from build123d import *

# Parameters (mm, degrees)
SKETCH_395_R           = 7.6
EXTRUDE_923_DEPTH      = 15
CUT_EXTRUDE_1359_DEPTH = 10
SKETCH_4236_W          = 30
SKETCH_4236_H          = 12
SKETCH_4236_R          = 2.15
SKETCH_4236_R_2        = 4.1
EXTRUDE_5757_DEPTH     = 15
SKETCH_1_3_R           = 12.15
SKETCH_1_3_R_2         = 10.65
CUT_EXTRUDE_5889_DEPTH = 5
SKETCH_1_4_R           = 10.65
CUT_EXTRUDE_5977_DEPTH = 8.5
CUT_EXTRUDE_7570_DEPTH = 6
SKETCH_1_R             = 7.65
EXTRUDE_7865_DEPTH     = 6.5


with BuildPart() as part:
    # Sketch 395 → Extrude 923 (new body)
    with BuildSketch(Plane.XY):
        with BuildLine():
            Line((33.023854242, 2.889212872), (32.0215632, 14.3454519))
            Line((32.0215632, 14.3454519), (35.508244643, 14.650497))
            Line((35.508244643, 14.650497), (33.329351075, 39.555364452))
            Line((33.329351075, 39.555364452), (56.241829131, 41.559946535))
            Line((56.241829131, 41.559946535), (58.4207227, 16.655079083))
            Line((58.4207227, 16.655079083), (61.907404143, 16.960124183))
            Line((61.907404143, 16.960124183), (62.909695184, 5.503885155))
            ThreePointArc((62.909695184, 5.503885155), (46.55906382, -42.663521611), (0, -63.15))
            ThreePointArc((0, -63.15), (-15, -48.15), (0, -33.15))
            ThreePointArc((0, -33.15), (24.440743715, -22.395815382), (33.023854242, 2.889212872))
        make_face()
        with Locations((0, -48.15)):
            Circle(SKETCH_395_R, mode=Mode.SUBTRACT)
    extrude(amount=EXTRUDE_923_DEPTH)

    # Sketch 978 → Cut-Extrude 1359 (cut)
    with BuildSketch(Plane(origin=(62.909695184, 5.503885155, 0), x_dir=(0, 0, -1), z_dir=(0.9961946980917458, 0.08715574274765542, 0))):
        with BuildLine():
            ThreePointArc((-6.5, 30), (-6.792893219, 30.707106781), (-7.5, 31))
            Line((-7.5, 31), (-7.5, 29))
            ThreePointArc((-7.5, 29), (-6.792893219, 29.292893219), (-6.5, 30))
        make_face()
        with BuildLine():
            Line((-7.5, 29), (-7.5, 31))
            ThreePointArc((-7.5, 31), (-8.5, 30), (-7.5, 29))
        make_face()
        with BuildLine():
            ThreePointArc((-6.5, 18), (-6.792893219, 18.707106781), (-7.5, 19))
            Line((-7.5, 19), (-7.5, 17))
            ThreePointArc((-7.5, 17), (-6.792893219, 17.292893219), (-6.5, 18))
        make_face()
        with BuildLine():
            Line((-7.5, 17), (-7.5, 19))
            ThreePointArc((-7.5, 19), (-8.5, 18), (-7.5, 17))
        make_face()
    cut_extrude_1359 = extrude(amount=-CUT_EXTRUDE_1359_DEPTH, mode=Mode.SUBTRACT)

    # Mirror 1435: Cut-Extrude 1359 across plane
    add(cut_extrude_1359.mirror(Plane(origin=(47.966774713, 4.196549013, 0), x_dir=(0, 0, 1), z_dir=(0.9961946980917455, 0.0871557427476578, 0))), mode=Mode.SUBTRACT)

    # Sketch 4236 → Extrude 5757 (add)
    # profile 1 of 5: a face of its own
    with BuildSketch(Plane(origin=(0, 0, 0), x_dir=(-1, 0, 0), z_dir=(0, 0, -1))):
        with BuildLine():
            ThreePointArc((0, -63.15), (-7.554244854, -62.69653806), (-15, -61.342664598))
            Line((-15, -61.342664598), (-15, -69.15))
            Line((-15, -69.15), (15, -69.15))
            Line((15, -69.15), (15, -48.15))
            ThreePointArc((15, -48.15), (10.606601718, -58.756601718), (0, -63.15))
        make_face()
    # profile 2 of 5: a face of its own
    with BuildSketch(Plane(origin=(0, 0, 0), x_dir=(-1, 0, 0), z_dir=(0, 0, -1))):
        with Locations((0, -75.15)):
            Rectangle(SKETCH_4236_W, SKETCH_4236_H)
        Polygon((-9.578460969, -72.55), (-5.421539031, -72.55), (-3.343078062, -76.15), (-5.421539031, -79.75), (-9.578460969, -79.75), (-11.656921938, -76.15), align=None, mode=Mode.SUBTRACT)
        Polygon((5.421539031, -79.75), (3.343078062, -76.15), (5.421539031, -72.55), (9.578460969, -72.55), (11.656921938, -76.15), (9.578460969, -79.75), align=None, mode=Mode.SUBTRACT)
    # profile 3 of 5: a face of its own
    with BuildSketch(Plane(origin=(0, 0, 0), x_dir=(-1, 0, 0), z_dir=(0, 0, -1))):
        Polygon((-5.421539031, -79.75), (-3.343078062, -76.15), (-5.421539031, -72.55), (-9.578460969, -72.55), (-11.656921938, -76.15), (-9.578460969, -79.75), align=None)
        with Locations((-7.5, -76.15)):
            Circle(SKETCH_4236_R, mode=Mode.SUBTRACT)
    # profile 4 of 5: a face of its own
    with BuildSketch(Plane(origin=(0, 0, 0), x_dir=(-1, 0, 0), z_dir=(0, 0, -1))):
        Polygon((5.421539031, -72.55), (9.578460969, -72.55), (11.656921938, -76.15), (9.578460969, -79.75), (5.421539031, -79.75), (3.343078062, -76.15), align=None)
        with Locations((7.5, -76.15)):
            Circle(SKETCH_4236_R, mode=Mode.SUBTRACT)
    # profile 5 of 5: a face of its own
    with BuildSketch(Plane(origin=(0, 0, 0), x_dir=(-1, 0, 0), z_dir=(0, 0, -1))):
        with Locations((0, -48.15)):
            Circle(SKETCH_4236_R_2)
    extrude(amount=-EXTRUDE_5757_DEPTH)


with BuildPart() as extrude_5757_kept_piece:
    # of the separate pieces the step leaves, the one the design keeps (extrude_5757_pieces_kept)
    add(part.part.solids().sort_by_distance((0, -33.15, 0))[0])

    # Эскиз1_3 → Cut-Extrude 5889 (cut)
    with BuildSketch(Plane(origin=(0, 0, 0), x_dir=(-1, 0, 0), z_dir=(0, 0, -1))):
        with Locations((0, -48.15)):
            Circle(SKETCH_1_3_R)
        with Locations((0, -48.15)):
            Circle(SKETCH_1_3_R_2, mode=Mode.SUBTRACT)
    extrude(amount=-CUT_EXTRUDE_5889_DEPTH, mode=Mode.SUBTRACT)

    # Эскиз1<4> → Cut-Extrude 5977 (cut)
    with BuildSketch(Plane(origin=(0, 0, 0), x_dir=(-1, 0, 0), z_dir=(0, 0, -1))):
        with Locations((0, -48.15)):
            Circle(SKETCH_1_4_R)
    extrude(amount=-CUT_EXTRUDE_5977_DEPTH, mode=Mode.SUBTRACT)

    # Sketch 6737 → Cut-Extrude 7570 (cut)
    with BuildSketch(Plane.XY.offset(15)):
        Polygon((5.421539031, -79.75), (3.343078062, -76.15), (5.421539031, -72.55), (9.578460969, -72.55), (11.656921938, -76.15), (9.578460969, -79.75), align=None)
        Polygon((-3.343078062, -76.15), (-5.421539031, -72.55), (-9.578460969, -72.55), (-11.656921938, -76.15), (-9.578460969, -79.75), (-5.421539031, -79.75), align=None)
    extrude(amount=-CUT_EXTRUDE_7570_DEPTH, mode=Mode.SUBTRACT)

    # Эскиз1 → Extrude 7865 (add)
    with BuildSketch(Plane(origin=(0, 0, 8.5), x_dir=(-1, 0, 0), z_dir=(0, 0, -1))):
        with Locations((0, -48.15)):
            Circle(SKETCH_1_R)
    extrude(amount=-EXTRUDE_7865_DEPTH)


solid = extrude_5757_kept_piece.part
Can you work these out from the model? Positions are in its coordinate system, mm. A direction names the side the tool comes from. Round coordinates to 2 decimals unless told otherwise and drop trailing zeros. Order: outer loops, then holes, each group sorted by start corner. A loop starts at its lowest first (then second) coordinate and runs counter-clockwise, first axis right, second up. Notation, with made-up numbers: M 43,46 L 66,46 A23 cw 66,84 Z; hole C 18.5,80 d3. An arc over 180 degrees is marked long. Use a Markdown table: item, result.
1) Imagine slicing it at A-A (z = 10.5). List the corners of the cut face in (x, y) for me.
Geometry says:
| item | result |
|---|---|
| outline | M -15,-81.15 L 15,-81.15 L 15,-61.34 A63.15 ccw 62.91,5.5 L 61.91,16.96 L 58.42,16.66 L 56.24,41.56 L 33.33,39.56 L 35.51,14.65 L 32.02,14.35 L 33.02,2.89 A33.15 cw 0,-33.15 A15 ccw -15,-48.15 Z; hole M -11.66,-76.15 L -9.58,-79.75 L -5.42,-79.75 L -3.34,-76.15 L -5.42,-72.55 L -9.58,-72.55 Z; hole M 3.34,-76.15 L 5.42,-79.75 L 9.58,-79.75 L 11.66,-76.15 L 9.58,-72.55 L 5.42,-72.55 Z |
2) I'm going to push flat-ended pins straight in: P1, Ø5, axis at y = 23.5, z = 3.5, coming from the -X side; P2, Ø5, axis at x = 41.5, z = 8.5, coming from the +Y side; P3, Ø2, axis at x = 41.5, z = 11.5, coming from the +Y side; P4, Ø4, axis at x = -7.5, y = -76.15, coming from the -Z side. Where does each tip first touch, or does it pass through?
Geometry says:
| item | result |
|---|---|
| P1 | stops at x = 34.52 |
| P2 | stops at y = 40.49 |
| P3 | stops at y = 40.36 |
| P4 | passes through |
3) Imagine slicing it at C-C (z = 3.5). List the corners of the cut face in (x, y) for me.
Geometry says:
| item | result |
|---|---|
| outline | M -15,-81.15 L 15,-81.15 L 15,-61.34 A63.15 ccw 62.91,5.5 L 61.91,16.96 L 58.42,16.66 L 56.24,41.56 L 33.33,39.56 L 35.51,14.65 L 32.02,14.35 L 33.02,2.89 A33.15 cw 0,-33.15 A15 ccw -15,-48.15 Z; hole C 0,-48.15 d24.3; hole C -7.5,-76.15 d4.3; hole C 7.5,-76.15 d4.3 |
4) On a 3-axis mill with a long thin cutter (end or side, diameter ignored), from which of +Z, -Z, +X, -X, +Y, -Y can I reach the whole of each face in a straight line? I mean faces 1 (the face through (15, -71, 7)), 2 (the face through (-11.59, -44.5, 2.46)), 3 (the face through (32.53, 8.54, 7.4)), 4 (the face through (-8, -79.75, 12)), 5 (the face through (-8.49, -78.06, 4.44)). Say none if no direction works.
Geometry says:
| item | result |
|---|---|
| face 1 | +Z, -Z, +X, -Y |
| face 2 | -Z |
| face 3 | +Z, -Z, -X |
| face 4 | +Z |
| face 5 | +Z, -Z |
5) Imagine slicing it at B-B (x = -7.5). List the corners of the cut face in (y, z) for me.
Geometry says:
| item | result |
|---|---|
| outline | M -81.15,0 L -78.3,0 L -78.3,9 L -79.75,9 L -79.75,15 L -81.15,15 Z; M -74,0 L -57.71,0 L -57.71,5 L -55.71,5 L -55.71,8.5 L -40.59,8.5 L -40.59,5 L -38.59,5 L -38.59,0 L -35.16,0 L -35.16,15 L -72.55,15 L -72.55,9 L -74,9 Z |
6) Imagine slicing it at D-D (y = -43). List the corners of the cut face in (x, z) for me, then the cut area to 3 significant figures.
Geometry says:
| item | result |
|---|---|
| outline | M -14.09,0 L -11,0 L -11,5 L -9.32,5 L -9.32,8.5 L 9.32,8.5 L 9.32,5 L 11,5 L 11,0 L 46.25,0 L 46.25,15 L -14.09,15 Z |
| area | 730 mm² |
7) If we mould it in two halves opening along Y, with no side actions, what happens to faces 6 (the face through (0, -48, 8.5)), 7 (the face through (62.4, 11.31, 7.4)), 8 (the face through (33, -19, 15)), 9 (the face through (8, -79.75, 12))? For each: +Y half, -Y half, draft (parallel to the pull), parting line (faces both ways), or undercut.
Geometry says:
| item | result |
|---|---|
| face 6 | undercut |
| face 7 | +Y half |
| face 8 | draft |
| face 9 | undercut |
8) If I drill on line 1 along Y through (x, z) = (-7.5, 6); line 2 along Y through (x, z) = (7.5, 6); line 3 along Y through (x, z) = (5, 13.25), over which ranges is the centre line in solid material (lowest first)?
Geometry says:
| item | result |
|---|---|
| line 1 | y = -81.15 to -78.3, -74 to -55.71, -40.59 to -35.16 |
| line 2 | y = -81.15 to -78.3, -74 to -55.71, -40.59 to -32.29 |
| line 3 | y = -81.15 to -79.02, -73.28 to -32.77 |
